from build123d import *

# Parameters (mm, degrees)
SKETCH1_W           = 120
SKETCH1_H           = 227
BOSS_EXTRUDE1_DEPTH = 2
SKETCH2_W           = 10
SKETCH2_H           = 2
BOSS_EXTRUDE2_DEPTH = 3
LPATTERN1_COUNT     = 5
LPATTERN1_PITCH     = 20
SKETCH3_W           = 10
SKETCH3_H           = 2
BOSS_EXTRUDE3_DEPTH = 3
LPATTERN2_COUNT     = 5
LPATTERN2_PITCH     = 20
SKETCH4_W           = 3
SKETCH4_H           = 10
CUT_EXTRUDE1_DEPTH  = 3
LPATTERN3_COUNT     = 11
LPATTERN3_PITCH     = 20
ESQUISSE1_W         = 1
ESQUISSE1_H         = 210
BOSS_EXTRU_1_DEPTH  = 2
ESQUISSE2_W         = 120
ESQUISSE2_H         = 1
BOSS_EXTRU_2_DEPTH  = 2


with BuildPart() as part:
    # Sketch1 → Boss-Extrude1 (new body)
    with BuildSketch(Plane(origin=(0, 0, 0), x_dir=(1, 0, 0), z_dir=(0, 1, 0))):
        with Locations((60, 113.5)):
            Rectangle(SKETCH1_W, SKETCH1_H)
    extrude(amount=BOSS_EXTRUDE1_DEPTH)

    # Sketch2 → Boss-Extrude2 (add)
    with BuildSketch(Plane.XY):
        with Locations((20, 1)):
            Rectangle(SKETCH2_W, SKETCH2_H)
    boss_extrude2 = extrude(amount=BOSS_EXTRUDE2_DEPTH)

    # LPattern1: Boss-Extrude2 ×5
    with Locations(*[(i * LPATTERN1_PITCH, 0, 0) for i in range(1, LPATTERN1_COUNT)]):
        add(boss_extrude2)

    # Sketch3 → Boss-Extrude3 (add)
    with BuildSketch(Plane(origin=(0, 0, -227), x_dir=(-1, 0, 0), z_dir=(0, 0, -1))):
        with Locations((-100, 1)):
            Rectangle(SKETCH3_W, SKETCH3_H)
    boss_extrude3 = extrude(amount=BOSS_EXTRUDE3_DEPTH)

    # LPattern2: Boss-Extrude3 ×5
    with Locations(*[(-i * LPATTERN2_PITCH, 0, 0) for i in range(1, LPATTERN2_COUNT)]):
        add(boss_extrude3)

    # Sketch4 → Cut-Extrude1 (cut, through all)
    with BuildSketch(Plane(origin=(0, 2, 0), x_dir=(1, 0, 0), z_dir=(0, 1, 0))):
        with Locations((21.5, 15)):
            Rectangle(SKETCH4_W, SKETCH4_H)
    cut_extrude1 = extrude(amount=-CUT_EXTRUDE1_DEPTH, mode=Mode.SUBTRACT)

    # LPattern3: Cut-Extrude1 ×11
    with Locations(*[(0, 0, -i * LPATTERN3_PITCH) for i in range(1, LPATTERN3_COUNT)]):
        add(cut_extrude1, mode=Mode.SUBTRACT)

    # Esquisse1 → Boss.-Extru.1 (add)
    with BuildSketch(Plane(origin=(0, 2, 0), x_dir=(1, 0, 0), z_dir=(0, 1, 0))):
        with Locations((22.5, 115)):
            Rectangle(ESQUISSE1_W, ESQUISSE1_H)
    extrude(amount=-BOSS_EXTRU_1_DEPTH)

    # Esquisse2 → Boss.-Extru.2 (add)
    with BuildSketch(Plane.XZ):
        with Locations((60, 0.5)):
            Rectangle(ESQUISSE2_W, ESQUISSE2_H)
    extrude(amount=-BOSS_EXTRU_2_DEPTH)


solid = part.part
Part model, mm, in its own coordinate system. Round coordinates to 2 decimals unless told otherwise and drop trailing zeros. Write each loop counter-clockwise with the first axis right and the second up, starting at its lowest first coordinate (ties: lowest second). Pieces come first, ordered by that corner, then holes. Notation, with made-up numbers: M 3,43 L 33,43 A32 ccw 33,80 Z; hole C -25,13.25 d8. An arc over 180 degrees is marked long. Return JSON: item names as keys, results as strings. Group by question number.
(1) Drill centre lines: probe 1 along X at (y, z) = (0.75, -118.5); probe 2 along Z at (x, y) = (11, 1.6). Where is each one in solid material? Low to high.
(2) Pin check, flat tips, straight feed: pin 1 Ø1 at (y, z) = (1, -15.5) entering from -X; pin 2 Ø1 at (x, y) = (50, 0.5) entering from -Z; pin 3 Ø0.6 at (y, z) = (1, -228.5) entering from -X. Stop position of each tip, or through.
(3) Saw through at C-C on x = 109. Write the cut outline in (y, z).
(4) Saw through at A-A on z = -16. Write the cut outline in (x, y), then the cut area to 3 significant figures.
(5) Saw through at B-B on y = 1.35. Count the separate pieces of the cut face and the enclosed holes in it, then the cut area to 3 significant figures.
Returned:
{
 "1": {"probe 1": "0 to 20, 22 to 120", "probe 2": "-227 to 1"},
 "2": {"pin 1": "x = 0", "pin 2": "z = -227", "pin 3": "x = 15"},
 "3": {"outline": "M 0,-227 L 2,-227 L 2,1 L 0,1 Z"},
 "4": {"outline": "M 0,0 L 20,0 L 20,2 L 0,2 Z; M 22,0 L 120,0 L 120,2 L 22,2 Z", "area": "236 mm²"},
 "5": {"separate pieces": "1", "enclosed holes": "11", "area": "27,400 mm²"}
}
